CAD build for the part. Positions are in the model's coordinates, mm. A direction names the side the tool comes from. Give positions to 0.01 mm unless a question says otherwise; leave off trailing zeros. Order: outer loops, then holes, each group sorted by start corner. A loop starts at its lowest first (then second) coordinate and runs counter-clockwise, first axis right, second up. Notation, with made-up numbers: (66.5, -27.75) -> (71.5, -27.75) arc R8 cw to (71.5, -12.75) -> close; hole circle Ø5 at (55.5, 50). An arc over 180 degrees is marked (long way). Answer as CSV lines item,"result".
```python
from build123d import *

# Parameters (mm, degrees)
F1_DEPTH = 15
F2_R     = 1.5
F3_DEPTH = 25
F4_R     = 1.5
F5_DEPTH = 25


with BuildPart() as f1:
    # F0 (on Top) → F1 (new body)
    with BuildSketch(Plane.XY):
        with BuildLine():
            ThreePointArc((24.306717, -1.304678), (15.502635, -0.15397), (24.207405, 1.596164))
            Line((24.207405, 1.596164), (29.928384, 1.596164))
            Line((29.928384, 1.596164), (29.928384, 4.922138))
            Line((29.928384, 4.922138), (23.431116, 4.922138))
            ThreePointArc((23.431116, 4.922138), (17.916276, 5.626553), (14.190525, 1.5))
            Line((14.190525, 1.5), (11.973724, 1.5))
            Line((11.973724, 1.5), (0, 1.5))
            Line((0, 1.5), (0, 0))
            Line((0, 0), (0, -1.5))
            Line((0, -1.5), (0, -1.8))
            Line((0, -1.8), (11.019785, -1.8))
            Line((11.019785, -1.8), (14.276365, -1.8))
            ThreePointArc((14.276365, -1.8), (18.063289, -5.678834), (23.431116, -4.922138))
            Line((23.431116, -4.922138), (29.928384, -4.922138))
            Line((29.928384, -4.922138), (29.928384, -1.304678))
            Line((29.928384, -1.304678), (24.306717, -1.304678))
        make_face()
    extrude(amount=F1_DEPTH)

    # F2 (on face) → F3 (cut)
    with BuildSketch(Plane.XZ.offset(1.8)):
        with Locations((5, 10)):
            Circle(F2_R)
    extrude(amount=-F3_DEPTH, mode=Mode.SUBTRACT)

    # F4 (on face) → F5 (cut)
    with BuildSketch(Plane.XZ.offset(4.922138)):
        with Locations((27.428384, 7.5)):
            Circle(F4_R)
    extrude(amount=-F5_DEPTH, mode=Mode.SUBTRACT)


solid = f1.part
```
1) Band-saw the part on B-B, the plane x = 20. Write the cut outline in (y, z).
Data:
outline,"(-6, 0) -> (-4.5, 0) -> (-4.5, 15) -> (-6, 15) -> close; (4.5, 0) -> (6, 0) -> (6, 15) -> (4.5, 15) -> close"
2) Band-saw the part on A-A, the plane z = 10. Write the cut outline in (x, y), then the cut area to 3 significant figures.
Data:
outline,"(0, -1.8) -> (3.5, -1.8) -> (3.5, 1.5) -> (0, 1.5) -> close; (6.5, -1.8) -> (14.28, -1.8) arc R6 ccw to (23.43, -4.92) -> (29.93, -4.92) -> (29.93, -1.3) -> (24.31, -1.3) arc R4.5 cw (long way) to (24.21, 1.6) -> (29.93, 1.6) -> (29.93, 4.92) -> (23.43, 4.92) arc R6 ccw to (14.19, 1.5) -> (6.5, 1.5) -> close"
area,"116 mm2"
3) Pull direction Y, two halves, no side cores. Call faces 4 (the flat face through (27.2, -1.305, 5.7)), 5 (the flat face through (25, 4.922, 7)), 6 (the flat face through (0, 0, 7)): pulls with the +Y half, pulls with the -Y half, needs draft (parallel to the pull), parting line crosses it, or undercut.
Data:
face 4,"undercut"
face 5,"pulls with the +Y half"
face 6,"needs draft"
4) Band-saw the part on C-C, the plane y = -3. Write the cut outline in (x, z).
Data:
outline,"(14.8, 0) -> (16.65, 0) -> (16.65, 15) -> (14.8, 15) -> close; (23.35, 0) -> (29.93, 0) -> (29.93, 15) -> (23.35, 15) -> close; hole circle Ø3 at (27.43, 7.5)"
5) Pin check, flat tips, straight feed: P1, Ø3, axis at x = 25, z = 6, coming from the +Y side; P2, Ø2, axis at y = 3, z = 2, coming from the -X side; P3, Ø8, axis at x = 3, z = 2, coming from the -Y side. Stop position of each tip, or through.
Data:
P1,"stops at y = 4.92"
P2,"stops at x = 14.34"
P3,"stops at y = -1.8"
6) Wall check: line 1 along Y through (x, z) = (25.5, 12.25); line 2 along Y through (x, z) = (19.75, 11.5); line 3 along Y through (x, z) = (14, 12). Give the ranges that are in metal, low to high. Write a range as [from, to].
Data:
line 1,"y = [-4.92, -1.3], [1.6, 4.92]"
line 2,"y = [-5.99, -4.49], [4.49, 5.99]"
line 3,"y = [-1.8, 1.5]"
7) Which spindle directions (+Z, -Z, +X, -X, +Y, -Y) get a long thin tool onto all of the face, cutting with end or side? Do faces 1 (the flat face through (7, -1.8, 7)), 2 (the flat face through (25, -4.922, 7)), 3 (the flat face through (7, 1.5, 7)). Say none if no direction does.
Data:
face 1,"+Z, -Z, -X, -Y"
face 2,"+Z, -Z, +X, -Y"
face 3,"+Z, -Z, -X, +Y"
8) Band-saw the part on D-D, the plane z = 7.5. Write the cut outline in (x, y), then the cut area to 3 significant figures.
Data:
outline,"(0, -1.8) -> (14.28, -1.8) arc R6 ccw to (23.43, -4.92) -> (25.93, -4.92) -> (25.93, -1.3) -> (24.31, -1.3) arc R4.5 cw (long way) to (24.21, 1.6) -> (25.93, 1.6) -> (25.93, 4.92) -> (23.43, 4.92) arc R6 ccw to (14.19, 1.5) -> (0, 1.5) -> close; (28.93, -4.92) -> (29.93, -4.92) -> (29.93, -1.3) -> (28.93, -1.3) -> close; (28.93, 1.6) -> (29.93, 1.6) -> (29.93, 4.92) -> (28.93, 4.92) -> close"
area,"105 mm2"
